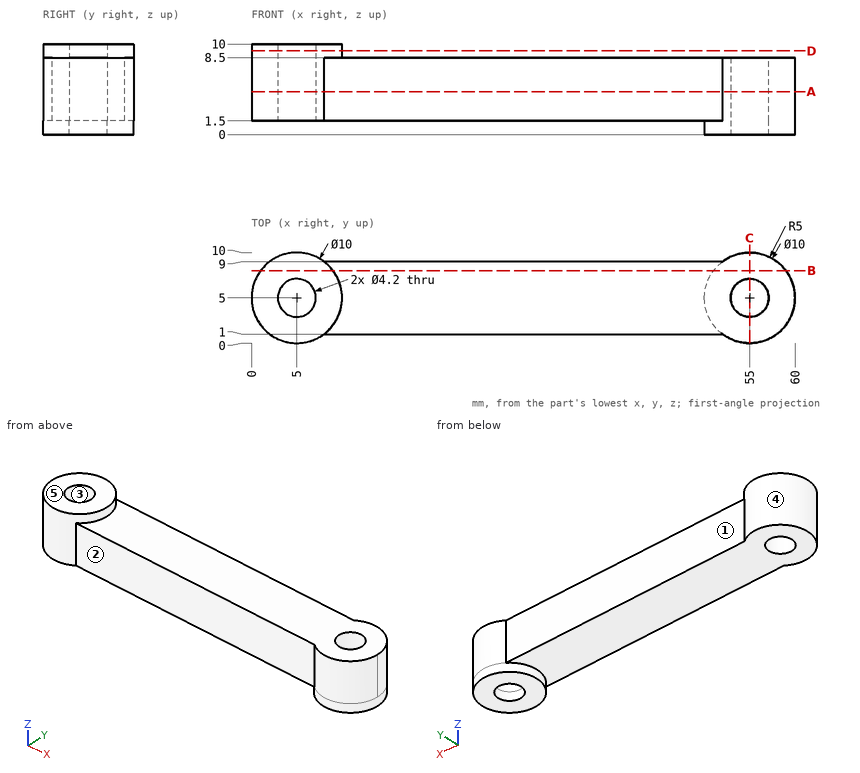
Study the drawing (mm; zero at the part's minimum x, y, z) and answer. A direction names the side the tool comes from. Coordinates: 2 decimals unless noted, no trailing zeros. Write each loop counter-clockwise with the first axis right and the second up, starting at its lowest first coordinate (ties: lowest second). Pieces come first, ordered by that corner, then holes. Notation, with made-up numbers: (69.25, -19) -> (82.25, -19) arc R19 cw to (82.25, 1) -> close; hole circle Ø9 at (0.25, -40). An arc over 180 degrees is marked (long way). Write each question's results on one line, items separated by ' | '. Start each with the question number.
1) A tool of negligible diameter and unlimited length cuts with its end or side. For the marked faces 1, 2 and 3, from which of +Z, -Z, +X, -X, +Y, -Y can it reach the whole face along a straight path? Write none if from no direction.
2) A cutting plane is placed at A-A (z = 4.75). Determine the outline of the cut face in (x, y).
3) A cutting plane is placed at C-C (x = 55). Determine the outline of the cut face in (y, z).
4) Straight lines are drawn through the part: probe 1 along Y at (x, z) = (5, 5); probe 2 along Z at (x, y) = (16, 1.75); probe 3 along Y at (x, z) = (30.5, 2.75). For each, find the intervals that lie inside material, in ascending order.
5) Flat-ended cylindrical pins translate along their axes: pin 1 Ø1 at (y, z) = (1.5, 2.5) entering from +X; pin 2 Ø1 at (x, z) = (35, 8.5) entering from -Y; pin 3 Ø5 at (x, z) = (20.5, 6) entering from +Y. Find the tip coordinate at first contact, or state that the pin passes through.
6) For a pull along X with two mould halves and no side action, classify the marked faces 4 and 5 as +X half, -X half, draft (parallel to the pull), parting line (faces both ways), or undercut.
7) A cutting plane is placed at D-D (z = 9.25). Determine the outline of the cut face in (x, y).
8) A cutting plane is placed at B-B (y = 8). Determine the outline of the cut face in (x, z).
Values follow:
1) face 1: +Z, -Z, +Y | face 2: +Z, -Z, -Y | face 3: +Z, -Z
2) outline: (8, 1) -> (52, 1) arc R5 ccw (long way) to (52, 9) -> (8, 9) arc R5 ccw (long way) to start; hole circle Ø4.2 at (5, 5); hole circle Ø4.2 at (55, 5)
3) outline: (0, 0) -> (2.9, 0) -> (2.9, 8.5) -> (0, 8.5) -> close; (7.1, 0) -> (10, 0) -> (10, 8.5) -> (7.1, 8.5) -> close
4) probe 1: 0 to 2.9, 7.1 to 10 | probe 2: 1.5 to 8.5 | probe 3: 1 to 9
5) pin 1: x = 59 | pin 2: y = 1 | pin 3: y = 9
6) face 4: undercut | face 5: draft
7) outline: circle Ø10 at (5, 5); hole circle Ø4.2 at (5, 5)
8) outline: (1, 1.5) -> (51, 1.5) -> (51, 0) -> (59, 0) -> (59, 8.5) -> (9, 8.5) -> (9, 10) -> (1, 10) -> close
